```python
from build123d import *

# Parameters (mm, degrees)
F0_R     = 2.1
F1_DEPTH = 5
F2_DEPTH = 25


with BuildPart() as f1:
    # F0 (on Top) → F1 (new body)
    with BuildSketch(Plane.XY):
        with BuildLine():
            ThreePointArc((-16.535554, -15.320309), (-18.755721, -12.504373), (-20.501266, -9.372007))
            ThreePointArc((-20.501266, -9.372007), (-21.062104, -8.032695), (-21.535554, -6.660055))
            Line((-21.535554, -6.660055), (-41.229833, -18.030553))
            ThreePointArc((-41.229833, -18.030553), (-38.971143, -22.5), (-36.229833, -26.690807))
            Line((-36.229833, -26.690807), (-16.535554, -15.320309))
        make_face()
        with BuildLine():
            Line((-5, 44.72136), (-5, 21.980364))
            ThreePointArc((-5, 21.980364), (0, 22.541881), (5, 21.980364))
            Line((5, 21.980364), (5, 44.72136))
            ThreePointArc((5, 44.72136), (0, 45), (-5, 44.72136))
        make_face()
        with BuildLine():
            ThreePointArc((21.535554, -6.660055), (21.062104, -8.032695), (20.501266, -9.372007))
            ThreePointArc((20.501266, -9.372007), (18.755721, -12.504373), (16.535554, -15.320309))
            Line((16.535554, -15.320309), (36.229833, -26.690807))
            ThreePointArc((36.229833, -26.690807), (38.971143, -22.5), (41.229833, -18.030553))
            Line((41.229833, -18.030553), (21.535554, -6.660055))
        make_face()
        with BuildLine():
            ThreePointArc((-20.501266, -9.372007), (-18.872007, -4.998734), (-14.498734, -6.627993))
            ThreePointArc((-14.498734, -6.627993), (-3.391643, 15.576917), (15.941881, 0))
            ThreePointArc((15.941881, 0), (15.576917, -3.391643), (14.498734, -6.627993))
            ThreePointArc((14.498734, -6.627993), (18.202077, -4.775548), (20.8, -8))
            ThreePointArc((20.8, -8), (20.724452, -8.702077), (20.501266, -9.372007))
            ThreePointArc((20.501266, -9.372007), (21.062104, -8.032695), (21.535554, -6.660055))
            ThreePointArc((21.535554, -6.660055), (22.28888, -3.367827), (22.541881, 0))
            ThreePointArc((22.541881, 0), (17.618823, 14.061063), (5, 21.980364))
            ThreePointArc((5, 21.980364), (0, 22.541881), (-5, 21.980364))
            ThreePointArc((-5, 21.980364), (-19.521842, 11.270941), (-21.535554, -6.660055))
            ThreePointArc((-21.535554, -6.660055), (-21.062104, -8.032695), (-20.501266, -9.372007))
        make_face()
        with BuildLine():
            ThreePointArc((20.8, -8), (18.202077, -4.775548), (14.498734, -6.627993))
            ThreePointArc((14.498734, -6.627993), (16.127993, -11.001266), (20.501266, -9.372007))
            ThreePointArc((20.501266, -9.372007), (20.724452, -8.702077), (20.8, -8))
        make_face()
        with Locations((17.5, -8)):
            Circle(F0_R, mode=Mode.SUBTRACT)
        with Locations((17.5, -8)):
            Circle(F0_R)
        with BuildLine():
            ThreePointArc((-14.498734, -6.627993), (-14.275548, -7.297923), (-14.2, -8))
            ThreePointArc((-14.2, -8), (-16.797924, -11.224452), (-20.501266, -9.372007))
            ThreePointArc((-20.501266, -9.372007), (-18.755721, -12.504373), (-16.535554, -15.320309))
            ThreePointArc((-16.535554, -15.320309), (0, -22.541881), (16.535554, -15.320309))
            ThreePointArc((16.535554, -15.320309), (18.755721, -12.504373), (20.501266, -9.372007))
            ThreePointArc((20.501266, -9.372007), (16.127993, -11.001266), (14.498734, -6.627993))
            ThreePointArc((14.498734, -6.627993), (0, -15.941881), (-14.498734, -6.627993))
        make_face()
        with BuildLine():
            ThreePointArc((-20.501266, -9.372007), (-16.797924, -11.224452), (-14.2, -8))
            ThreePointArc((-14.2, -8), (-14.275548, -7.297923), (-14.498734, -6.627993))
            ThreePointArc((-14.498734, -6.627993), (-18.872007, -4.998734), (-20.501266, -9.372007))
        make_face()
        with Locations((-17.5, -8)):
            Circle(F0_R, mode=Mode.SUBTRACT)
        with Locations((-17.5, -8)):
            Circle(F0_R)
    extrude(amount=F1_DEPTH)

    # F0 (on Top) → F2 (join)
    with BuildSketch(Plane.XY):
        with BuildLine():
            ThreePointArc((-20.501266, -9.372007), (-16.797924, -11.224452), (-14.2, -8))
            ThreePointArc((-14.2, -8), (-14.275548, -7.297923), (-14.498734, -6.627993))
            ThreePointArc((-14.498734, -6.627993), (-18.872007, -4.998734), (-20.501266, -9.372007))
        make_face()
        with Locations((-17.5, -8)):
            Circle(F0_R, mode=Mode.SUBTRACT)
        with BuildLine():
            ThreePointArc((20.8, -8), (18.202077, -4.775548), (14.498734, -6.627993))
            ThreePointArc((14.498734, -6.627993), (16.127993, -11.001266), (20.501266, -9.372007))
            ThreePointArc((20.501266, -9.372007), (20.724452, -8.702077), (20.8, -8))
        make_face()
        with Locations((17.5, -8)):
            Circle(F0_R, mode=Mode.SUBTRACT)
    extrude(amount=F2_DEPTH)


solid = f1.part
```
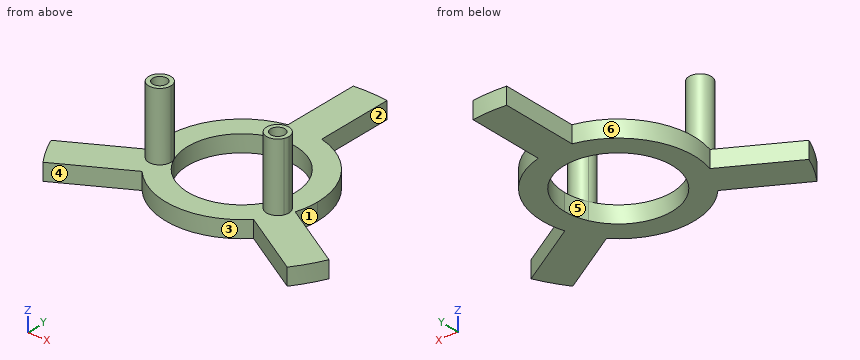
Check sheet for the modelled part. Datum: model origin and axes. Units: mm. Face numbers are marked on the shaded views. A direction names the side the tool comes from. Give positions to 0.01 mm unless a question says otherwise; leave off trailing zeros. Write each loop counter-clockwise with the first axis right and the second up, starting at its lowest first coordinate (ties: lowest second). Pieces come first, ordered by that corner, then holes.
Item 1: Scan lines: L1, parallel to X at y = -8, z = 12.5; L2, parallel to Y at x = -17.5, z = 12.75; L3, parallel to X at y = 32, z = 1.25. Record each from-to range of solid material in increasing order.
Item 2: Cross-section at D-D (x = -17.5). Enter the section's corners in (y, z).
Item 3: Cross-section at C-C (y = -3.5). Enter the section's corners in (x, z).
Item 4: Cross-section at A-A (z = 6.5). Enter the section's corners in (x, y), and give its area (3 significant figures).
Item 5: Cross-section at B-B (x = 0). Enter the section's corners in (y, z), and give its area (3 significant figures).
Item 6: Gauge pin test, flat ends, axial feed: pin 1 (4 mm diameter, centred on y = 32.5, z = 3, fed in from +X); pin 2 (12 mm diameter, centred on x = -31.5, z = 12.5, fed in from +Y); pin 3 (5.5 mm diameter, centred on x = -17.5, y = -8, fed in from +Z); pin 4 (4 mm diameter, centred on y = 36, z = 3, fed in from -X). Record the tip position at first contact, or that the pin passes through.
Item 7: Access from +Z, -Z, +X, -X, +Y, -Y to the whole of each face (thin tool, end or side, straight path). Record for the marked faces 4, 5 and 6.
Item 8: Draft check along Y on the marked faces 1, 2 and 3. Enter one of: released by +Y, released by -Y, zero draft, split by the parting line, or undercut.
Report:
1. L1: x = -20.8 to -19.6, -15.4 to -14.2, 14.2 to 15.4, 19.6 to 20.8
1. L2: y = -11.3 to -10.1, -5.9 to -4.7
1. L3: x = -5 to 5
2. outline: (-15.88, 0) - (14.21, 0) - (14.21, 5) - (-4.7, 5) - (-4.7, 25) - (-5.9, 25) - (-5.9, 5) - (-10.1, 5) - (-10.1, 25) - (-11.3, 25) - (-11.3, 5) - (-15.88, 5) - close
3. outline: (-22.27, 0) - (-15.55, 0) - (-15.55, 5) - (-22.27, 5) - close; (15.55, 0) - (22.27, 0) - (22.27, 5) - (15.55, 5) - close
4. outline: (-14.5, -6.63) arc R3.3 ccw (long way) to (-14.2, -8) arc R3.3 ccw to start; (20.5, -9.37) arc R3.3 ccw to (20.8, -8) arc R3.3 ccw (long way) to start; hole circle Ø4.2 at (-17.5, -8); hole circle Ø4.2 at (17.5, -8)
4. area: 40.7 mm2
5. outline: (-22.54, 0) - (-15.94, 0) - (-15.94, 5) - (-22.54, 5) - close; (15.94, 0) - (45, 0) - (45, 5) - (15.94, 5) - close
5. area: 178 mm2
6. pin 1: stops at x = 5
6. pin 2: passes through
6. pin 3: stops at z = 25
6. pin 4: stops at x = -5
7. face 4: +Z, -Z, -Y
7. face 5: +Z, -Z
7. face 6: +Z, -Z, -X
8. face 1: undercut
8. face 2: zero draft
8. face 3: released by -Y
